Could you check a few things on this drawing? It's one solid part, dimensions in mm from its lowest x, y, z. A direction names the side the tool comes from. Give positions to 0.01 mm unless a question says otherwise; leave off trailing zeros. Loops run counter-clockwise (first coordinate to the right, second up) from the corner with the lowest first, then second, coordinate; pieces in that order, holes last. Notation, with made-up numbers: M 11.25,53 L 60.25,53 A22 ccw 60.25,84 Z; hole C -11,76.25 d6. An arc over 180 degrees is marked long. Answer in a Markdown table with one row per item. Add a question column.
1. If we section it at D-D on z = 4.25: List the corners of the cut face in (x, y) for me.
2. If we section it at B-B on y = 4.5: List the corners of the cut face in (x, z) for me.
3. I'm going to push flat-ended pins straight in: pin 1 Ø6 at (x, y) = (35.5, 17) entering from -Z; pin 2 Ø1.5 at (x, z) = (25.5, 14.5) entering from -Y; pin 3 Ø6.5 at (x, y) = (22, 4.5) entering from +Z. Where does each tip first touch, or does it pass through?
4. Which directions (+Z, -Z, +X, -X, +Y, -Y) give clear straight access to the entire face, cutting with the end or side of a thin tool? Please do the marked faces 1, 2 and 3.
5. I need wall thicknesses on line 1 along Y through (x, z) = (22, 18.2); line 2 along Z through (x, y) = (3, 17.5); line 3 along Z through (x, y) = (18.5, 17.5). Which ranges of each line are inside material? Lowest first, please. Write a range as from..to.
6. If we section it at A-A on y = 22: List the corners of the cut face in (x, z) for me, then the cut area to 3 significant figures.
7. If we section it at C-C on x = 27: List the corners of the cut face in (y, z) for me (1 decimal), then the cut area to 3 significant figures.
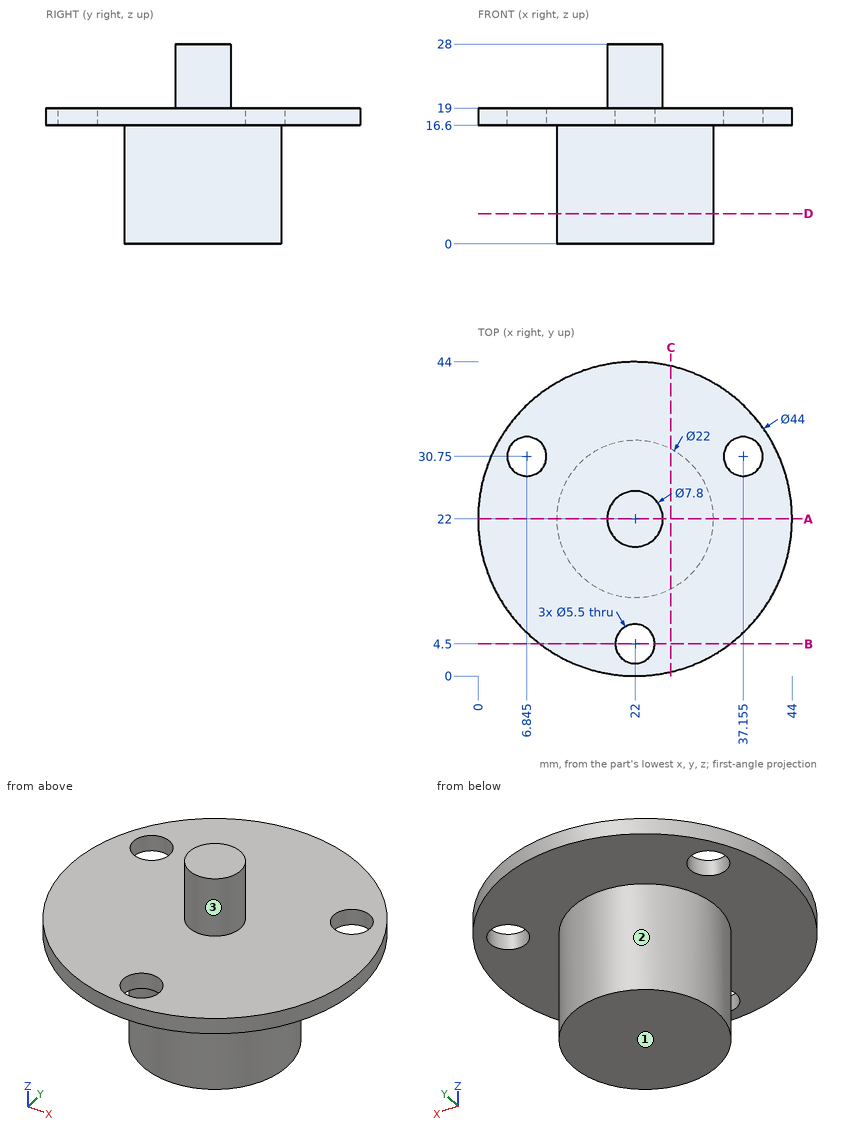
Results:
| question | item | result |
|---|---|---|
| 1 | outline | C 22,22 d22 |
| 2 | outline | M 8.67,16.6 L 19.25,16.6 L 19.25,19 L 8.67,19 Z; M 24.75,16.6 L 35.33,16.6 L 35.33,19 L 24.75,19 Z |
| 3 | pin 1 | z = 16.6 |
| 3 | pin 2 | y = 11.35 |
| 3 | pin 3 | z = 19 |
| 4 | face 1 | -Z, +X, -X, +Y, -Y |
| 4 | face 2 | -Z |
| 4 | face 3 | +Z |
| 5 | line 1 | 0..1.75, 7.25..44 |
| 5 | line 2 | 16.6..19 |
| 5 | line 3 | 0..19 |
| 6 | outline | M 0,16.6 L 11,16.6 L 11,0 L 33,0 L 33,16.6 L 44,16.6 L 44,19 L 25.9,19 L 25.9,28 L 18.1,28 L 18.1,19 L 0,19 Z |
| 6 | area | 541 mm2 |
| 7 | outline | M 0.6,16.6 L 12.2,16.6 L 12.2,0 L 31.8,0 L 31.8,16.6 L 43.4,16.6 L 43.4,19 L 0.6,19 Z |
| 7 | area | 428 mm2 |
